CAD build for the part. Positions are in the model's coordinates, mm. A direction names the side the tool comes from. Round coordinates to 2 decimals unless told otherwise and drop trailing zeros. Loops run counter-clockwise (first coordinate to the right, second up) from the corner with the lowest first, then second, coordinate; pieces in that order, holes last. Notation, with made-up numbers: (27.25, -27.5) - (77.25, -27.5) arc R19 cw to (77.25, -9.5) - close; hole circle Ø8 at (41.5, 27.25). An arc over 180 degrees is marked (long way). Use one line per item in the form item = value.
Autodesk Inventor part; units mm, degrees
ref_plane "YZ Plane" through (0, 0, 0) normal (1, 0, 0) x (0, 1, 0)
ref_plane "XZ Plane" through (0, 0, 0) normal (0, 1, 0) x (-1, 0, 0)
ref_plane "XY Plane" through (0, 0, 0) normal (0, 0, 1) x (1, 0, 0)
ref_plane "Work Plane1" through (0, 0, 2) normal (0, 0, 1) x (1, 0, 0)
sketch "Sketch1" plane through (0, 0, 2) normal (0, 0, 1) x (1, 0, 0)
  circle A0 centre (-37.0712, 14) radius 3.25 construction
  circle A1 centre (-9.0712, -14) radius 3.25 construction
  line L0 (-26.0712, -17.08) -> (-20.0712, -17.08) construction
  arc A2 (-20.0712, -17.08) -> (-20.0712, -14.08) centre (-20.0712, -15.58) ccw construction
  line L1 (-20.0712, -14.08) -> (-26.0712, -14.08) construction
  line L2 (-37.0712, -3) -> (-37.0712, 3) construction
  arc A3 (-37.0712, 3) -> (-40.0712, 3) centre (-38.5712, 3) ccw construction
  line L3 (-40.0712, 3) -> (-40.0712, -3) construction
  line L4 (-47.9712, -17) -> (-47.9712, 17) construction
  line L5 (-47.9712, 17) -> (-44.3964, 17) construction
  line L6 (-44.3964, 17) -> (-40.0712, 21.3252) construction
  line L7 (-40.0712, 21.3252) -> (-40.0712, 24.9) construction
  line L8 (-40.0712, 24.9) -> (-6.0712, 24.9) construction
  line L9 (-6.0712, 24.9) -> (-6.0712, 21.3252) construction
  line L10 (-6.0712, 21.3252) -> (-1.746, 17) construction
  line L11 (-1.746, 17) -> (1.8288, 17) construction
  line L12 (1.8288, 17) -> (1.8288, -17) construction
  line L13 (1.8288, -17) -> (-1.746, -17) construction
  line L14 (-1.746, -17) -> (-6.1126, -21.3666) construction
  line L15 (-6.1126, -21.3666) -> (-6.1126, -24.9) construction
  line L16 (-6.1126, -24.9) -> (-40.0712, -24.9) construction
  circle A4 centre (-37.0712, -14) radius 3.25 construction
  circle A5 centre (-23.0712, 0) radius 12.45 construction
  circle A6 centre (-23.0712, 0) radius 12.7 construction
  line L17 (-37.0712, 14) -> (-9.0712, 14) construction
  line L18 (-9.0712, 14) -> (-9.0712, -14) construction
  line L19 (-9.0712, -14) -> (-37.0712, -14) construction
  line L20 (-37.0712, -14) -> (-37.0712, 14) construction
  line L21 (-4.0712, -19) -> (-4.0712, 19)
  line L22 (-4.0712, 19) -> (-42.0712, 19)
  line L23 (-42.0712, 19) -> (-42.0712, -19)
  line L24 (-42.0712, -19) -> (-4.0712, -19)
  circle A7 centre (-23.0712, 0) radius 12.8
  circle A8 centre (-23.0712, 0) radius 3.25
  line L25 (-40.0712, -24.9) -> (-40.0712, -21.3252)
  line L26 (-40.0712, -21.3252) -> (-44.3964, -17)
  line L27 (-44.3964, -17) -> (-47.9712, -17)
  arc A9 (-26.0712, -14.08) -> (-26.0712, -17.08) centre (-26.0712, -15.58) ccw
  arc A10 (-40.0712, -3) -> (-37.0712, -3) centre (-38.5712, -3) ccw
  circle A11 centre (-37.0712, -14) radius 3.25
  point P0 (0, 0)
  point P1 (-21.8762, -3.0223)
  point P2 (-25.9925, 1.4242)
  dimension "d0" = 5
  dimension "d1" = 0.1
extrude "Extrusion1" add sketch "Sketch1" along normal blind 6 contours L24 L23 L22 L21 | A7 | A11
sketch "Sketch2" plane through (0, 0, 2) normal (0, 0, -1) x (-1, 0, 0)
  circle A0 centre (23.0712, 0) radius 12.8
  circle A1 centre (23.0712, 0) radius 8.5824
  point P0 (0, 0)
extrude "Extrusion2" add sketch "Sketch2" against normal blind 0.5
sketch "Sketch3" plane through (0, 0, 2) normal (0, 0, -1) x (-1, 0, 0)
  circle A0 centre (9.0712, -14) radius 1.45 construction
  circle A1 centre (9.0712, -14) radius 2.45
  circle A2 centre (37.0712, -14) radius 1.45
  circle A3 centre (37.0712, -14) radius 1.95
  point P0 (0, 0)
  dimension "d8" = 1
  dimension "d10" = 0.5
sketch "Sketch5" plane through (0, 0, 2) normal (0, 0, -1) x (-1, 0, 0)
  arc A0 (20.0712, -14.08) -> (20.0712, -17.08) centre (20.0712, -15.58) ccw
  arc A1 (26.0712, -17.08) -> (26.0712, -14.08) centre (26.0712, -15.58) ccw
  line L0 (37.0712, 3) -> (37.0712, -3)
  arc A2 (37.0712, -3) -> (40.0712, -3) centre (38.5712, -3) ccw
  line L1 (40.0712, -3) -> (40.0712, 3)
  arc A3 (40.0712, 3) -> (37.0712, 3) centre (38.5712, 3) ccw
  line L2 (26.0712, -14.08) -> (20.0712, -14.08)
  arc A4 (20.0712, -14.08) -> (20.0712, -17.08) centre (20.0712, -15.58) ccw
  line L3 (20.0712, -17.08) -> (26.0712, -17.08)
  arc A5 (26.0712, -17.08) -> (26.0712, -14.08) centre (26.0712, -15.58) ccw
  circle A6 centre (37.0712, -14) radius 1.45
  circle A7 centre (23.0712, 0) radius 1.45
  circle A8 centre (9.0712, -14) radius 1.45
  circle A9 centre (37.0712, 14) radius 1.45
  line L4 (-1.8288, -17) -> (-1.8288, 17)
  line L5 (-1.8288, 17) -> (1.746, 17)
  line L6 (1.746, 17) -> (6.0712, 21.3252)
  line L7 (6.0712, 21.3252) -> (6.0712, 24.9)
  line L8 (6.0712, 24.9) -> (40.0712, 24.9)
  line L9 (40.0712, 24.9) -> (40.0712, 21.3252)
  line L10 (40.0712, 21.3252) -> (44.3964, 17)
  line L11 (44.3964, 17) -> (47.9712, 17)
  line L12 (47.9712, 17) -> (47.9712, -17)
  line L13 (44.3964, -17) -> (47.9712, -17)
  line L14 (40.0712, -21.3252) -> (44.3964, -17)
  line L15 (40.0712, -24.9) -> (40.0712, -21.3252)
  line L16 (6.1126, -24.9) -> (40.0712, -24.9)
  line L17 (6.1126, -24.9) -> (6.1126, -21.3666)
  line L18 (6.1126, -21.3666) -> (1.746, -17)
  line L19 (1.746, -17) -> (-1.8288, -17)
  point P0 (0, 0)
  point P1 (40.0712, -3)
extrude "Extrusion5" cut sketch "Sketch5" against normal blind 8 contours L2 A1 L3 A0 | A3 L1 A2 L0
sketch "Sketch6" plane through (-42.0712, -19, 8) normal (0, -1, 0) x (1, 0, 0)
  line L0 (0, -6) -> (38, -6)
  line L1 (38, -6) -> (38, 0)
  line L2 (0, 0) -> (38, 0)
  line L3 (0, -6) -> (0, 0)
  line L4 (31.8, 0) -> (31.8, 0)
  circle A0 centre (19, -3) radius 1.45
  point P0 (42.0712, -8)
  point P1 (4.5, 0)
  dimension "d34" = 2.9
extrude "Extrusion6" cut sketch "Sketch6" against normal blind 8 contours A0
pattern_circular "Circular Pattern1" count 2 over 90 about axis through (-23.0712, 0, 2) along (0, 0, -1) of "Extrusion6"
chamfer "Chamfer1" distance 3 angle 45 4 edges at (-42.0712, 19, 5) (-4.0712, 19, 5) (-4.0712, -19, 5) (-42.0712, -19, 5)
hole "Hole1" at (-37.0712, -14, 2) direction (0, 0, 1) diameter 4 depth 0.1 tip angle 115
sketch "Sketch4" plane through (-4.0712, -19, 2) normal (1, 0, 0) x (0, 0, -1)
  line L0 (2, 4.45) -> (6, 4.45)
  line L1 (2, 1.55) -> (6, 1.55)
  line L2 (0, 0) -> (0, 38)
  arc A0 (2, 19) -> (2, 19) centre (1.5, 4.4206) ccw
  line L3 (-1.3741, 5) -> (-0.1, 7)
  line L4 (-1.3741, 5) -> (-0.1, 3)
  line L5 (-0.1, 7) -> (0.6045, 7)
  line L6 (0.6045, 7) -> (0.6045, 3)
  line L7 (0.6045, 3) -> (-0.1, 3)
  line L8 (-0.1, 3) -> (-0.1, 7)
extrude "Extrusion4" cut sketch "Sketch4" against normal blind 8 contours L7 L8 L5 L2 | L2 L5 L6 L7 | L4 L3 L8
sketch "Skizze8" plane through (0, 0, 8) normal (0, 0, 1) x (1, 0, 0)
  line L0 (-39.0712, -19) -> (-42.0712, -16)
  line L1 (-39.0712, -19) -> (-7.0712, -19)
  line L2 (-4.0712, -16) -> (-7.0712, -19)
  line L3 (-4.0712, -16) -> (-4.0712, 16)
  line L4 (-7.0712, 19) -> (-4.0712, 16)
  line L5 (-7.0712, 19) -> (-39.0712, 19)
  line L6 (-42.0712, 16) -> (-39.0712, 19)
  line L7 (-42.0712, 16) -> (-42.0712, -16)
  arc A0 (-37.0712, 3) -> (-40.0712, 3) centre (-38.5712, 3) ccw
  line L8 (-37.0712, 3) -> (-37.0712, -3)
  arc A1 (-40.0712, -3) -> (-37.0712, -3) centre (-38.5712, -3) ccw
  line L9 (-40.0712, -3) -> (-40.0712, 3)
  line L10 (-20.0712, -17.08) -> (-26.0712, -17.08)
  arc A2 (-26.0712, -14.08) -> (-26.0712, -17.08) centre (-26.0712, -15.58) ccw
  line L11 (-26.0712, -14.08) -> (-20.0712, -14.08)
  arc A3 (-20.0712, -17.08) -> (-20.0712, -14.08) centre (-20.0712, -15.58) ccw
  circle A4 centre (-23.0712, 0) radius 3.25
  line L12 (-9.0712, -14) -> (-37.0712, -14)
  line L13 (-37.0712, -14) -> (-37.0712, 14)
  line L14 (-37.0712, 14) -> (-9.0712, 14)
  line L15 (-9.0712, 14) -> (-9.0712, -14)
  line L16 (-9.0712, -14) -> (-37.0712, 14) construction
  line L17 (-37.0712, -14) -> (-9.0712, 14) construction
  point P0 (0, 0)
extrude "Extrusion8" add sketch "Skizze8" along normal blind 2 contours L13 L14 L15 L12 L8
properties part number "20_Cube_Insert_Kinematic_Beautymirrormount_90_pro_v3"
1) Two-plate mould, pull along Y, no slides. Class faces 1 (the flat face through (-40.55, 17.52, 4.96)), 2 (the flat face through (-12.071, -14, 3)), 3 (the flat face through (-40.59, -17.48, 4.96)): +Y half, -Y half, draft (parallel to the pull), parting line (faces both ways), or undercut.
Report:
face_1 = +Y half
face_2 = undercut
face_3 = -Y half
2) Tool access for faces 4 (the cylindrical face through (-35.592, 0.314, 3.584)), 5 (the cylindrical face through (-38.6, 4.5, 5)), 6 (the cylindrical face through (-24.52, -12.56, 5.06)): list every direction of +Z, -Z, +X, -X, +Y, -Y with a clear straight run to the whole face (end or side of a thin tool).
Report:
face_4 = -X
face_5 = +Z, -Z
face_6 = -Y
3) Drill centre lines: probe 1 along Y at (x, z) = (-22, 3.75); probe 2 along X at (y, z) = (3, 7.75); probe 3 along Z at (x, y) = (-36, 0). Where is each one in solid material? Low to high.
Report:
probe_1 = -19 to -17.08, -14.08 to -3.07, 3.07 to 19
probe_2 = -42.07 to -40.07, -37.07 to -24.32, -21.82 to -4.07
probe_3 = 2 to 3.55, 6.45 to 10
4) Flat gauge pins, fed straight in: pin 1 (1.4 mm diameter, centred on y = 0.5, z = 5, fed in from -X); pin 2 (3 mm diameter, centred on x = -22.5, z = 4.5, fed in from -Y); pin 3 (1.5 mm diameter, centred on x = -27, y = 15, fed in from +Z); pin 4 (0.6 mm diameter, centred on x = -27, z = 9, fed in from +Y). Where does each tip first touch, or does it go through?
Report:
pin_1 = -34.07
pin_2 = -19
pin_3 = 8
pin_4 = 14
5) Slice it at D-D (y = 5). Write the cut outline in (x, z), plus the area to 3 significant figures.
Report:
outline = (-42.07, 2) - (-4.07, 2) - (-4.07, 8) - (-9.07, 8) - (-9.07, 10) - (-37.07, 10) - (-37.07, 8) - (-42.07, 8) - close
area = 284 mm^2
6) Slice it at B-B (z = 9.5). Write the cut outline in (x, y).
Report:
outline = (-37.07, -14) - (-9.07, -14) - (-9.07, 14) - (-37.07, 14) - close; hole circle Ø6.5 at (-23.07, 0)
7) Slice it at A-A (y = 0). Write the cut outline in (x, z), plus the area to 4 significant figures.
Report:
outline = (-42.07, 2) - (-40.07, 2) - (-40.07, 3.55) - (-42.07, 3.55) - close; (-42.07, 6.45) - (-40.07, 6.45) - (-40.07, 8) - (-42.07, 8) - close; (-37.07, 2) - (-26.32, 2) - (-26.32, 10) - (-37.07, 10) - (-37.07, 6.45) - (-34.07, 6.45) - (-34.07, 3.55) - (-37.07, 3.55) - close; (-19.82, 2) - (-4.07, 2) - (-4.07, 8) - (-9.07, 8) - (-9.07, 10) - (-19.82, 10) - close
area = 199.5 mm^2
8) Slice it at C-C (x = -31). Write the cut outline in (y, z), plus the area to 3 significant figures.
Report:
outline = (-19, 2) - (19, 2) - (19, 8) - (14, 8) - (14, 10) - (-14, 10) - (-14, 8) - (-19, 8) - close
area = 284 mm^2
